Input: dimensioned drawing with shaded views. Units: mm. Origin: part minimum x, y, z. Coordinates: 2 decimals unless noted, no trailing zeros. Loops run counter-clockwise (first coordinate to the right, second up) from the corner with the lowest first, then second, coordinate; pieces in that order, holes last. Notation, with made-up numbers: (82, -4.75) - (95, -4.75) arc R11 ccw to (95, 13.25) - close; hole circle Ø9 at (43.5, 73). An arc over 180 degrees is marked (long way). Write item = value, one per line. Start each with the question number.
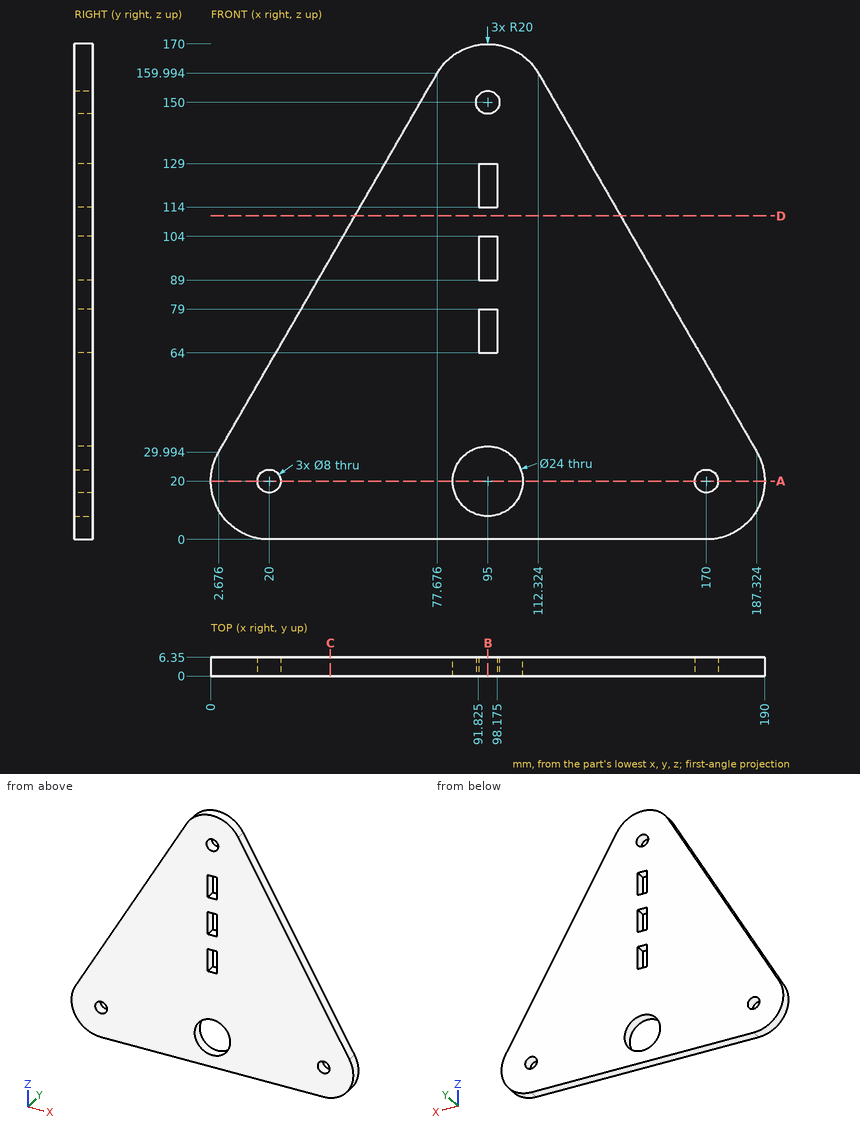
Item 1: Cut plane C-C on x = 41. Return loops of the section in (y, z).
Item 2: Cut plane D-D on z = 111. Return loops of the section in (x, y), plus the area to 3 significant figures.
Item 3: Ray query, line 1 (X direction, y = 2.5, z = 20); line 2 (Z direction, x = 97, y = 2.25) (1 decimal); line 3 (X direction, y = 0.75, z = 60). Return the intervals inside material, ascending.
Item 4: Cut plane B-B on x = 95. Return loops of the section in (y, z).
Item 5: Pin query (flat end, axial travel): pin 1 (2 mm diameter, centred on y = 4.5, z = 44.5, fed in from -X); pin 2 (3 mm diameter, centred on y = 1.5, z = 30, fed in from -X); pin 3 (1 mm diameter, centred on x = 134.5, y = 1.5, fed in from +Z) (1 decimal). Return the tip coordinate at first contact, or that it passes through.
Item 6: Cut plane A-A on z = 20. Return loops of the section in (x, y).
Recorded:
q1.outline = (0, 0) - (6.35, 0) - (6.35, 96.42) - (0, 96.42) - close
q2.outline = (49.41, 0) - (140.59, 0) - (140.59, 6.35) - (49.41, 6.35) - close
q2.area = 579 mm²
q3.line_1 = 0 to 16, 24 to 83, 107 to 166, 174 to 190
q3.line_2 = 0 to 8.2, 31.8 to 64, 79 to 89, 104 to 114, 129 to 146.5, 153.5 to 169.9
q3.line_3 = 19.99 to 170.01
q4.outline = (0, 0) - (6.35, 0) - (6.35, 8) - (0, 8) - close; (0, 32) - (6.35, 32) - (6.35, 64) - (0, 64) - close; (0, 79) - (6.35, 79) - (6.35, 89) - (0, 89) - close; (0, 104) - (6.35, 104) - (6.35, 114) - (0, 114) - close; (0, 129) - (6.35, 129) - (6.35, 146) - (0, 146) - close; (0, 154) - (6.35, 154) - (6.35, 170) - (0, 170) - close
q5.pin_1 = 10.47
q5.pin_2 = 1.9
q5.pin_3 = 122.4
q6.outline = (0, 0) - (16, 0) - (16, 6.35) - (0, 6.35) - close; (24, 0) - (83, 0) - (83, 6.35) - (24, 6.35) - close; (107, 0) - (166, 0) - (166, 6.35) - (107, 6.35) - close; (174, 0) - (190, 0) - (190, 6.35) - (174, 6.35) - close
